Verification items for the finished model (mm, model axes). A direction names the side the tool comes from. Round coordinates to 2 decimals unless told otherwise and drop trailing zeros. Loops run counter-clockwise (first coordinate to the right, second up) from the corner with the lowest first, then second, coordinate; pieces in that order, holes last. Notation, with made-up numbers: M 43.25,57 L 99.25,57 A32 cw 99.25,89 Z; hole C -25.75,-23.75 d4. An arc over 180 degrees is marked long. One line per item, written item: value.
from build123d import *

# Parameters (mm, degrees)
F0_R     = 5
F0_R_2   = 2.5
F1_DEPTH = 13
F0_R_3   = 7.5
F2_DEPTH = 3
F4_DEPTH = 3
F3_R     = 7.5
F3_R_2   = 5
F3_R_3   = 0.5
F5_DEPTH = 3
F6_R     = 1.425
F7_DEPTH = 25


with BuildPart() as f1:
    # F0 (on Front) → F1 (new body)
    with BuildSketch(Plane.XZ):
        Circle(F0_R)
        Circle(F0_R_2, mode=Mode.SUBTRACT)
    extrude(amount=F1_DEPTH)

    # F0 (on Front) → F2 (join)
    with BuildSketch(Plane.XZ):
        Circle(F0_R_3)
        Circle(F0_R, mode=Mode.SUBTRACT)
    extrude(amount=-F2_DEPTH)

    # F4 (add): a face of the model
    f4_faces = [f1.faces().sort_by_distance(p)[0] for p in [
        (-4.8585786438, 0, 0),
    ]]
    extrude(f4_faces, amount=F4_DEPTH)

    # F3 (on face) → F5 (join)
    with BuildSketch(Plane.XZ.offset(13)):
        Circle(F3_R)
        Circle(F3_R_2, mode=Mode.SUBTRACT)
        with Locations((5.9560983991, 0.7244942103)):
            Circle(F3_R_3, mode=Mode.SUBTRACT)
        with Locations((4.9608234595, 3.3749415703)):
            Circle(F3_R_3, mode=Mode.SUBTRACT)
    extrude(amount=-F5_DEPTH)

    # F6 (on Right) → F7 (cut)
    with BuildSketch(Plane.YZ):
        with Locations((-5, 0)):
            Circle(F6_R)
    extrude(amount=-F7_DEPTH, mode=Mode.SUBTRACT)


solid = f1.part
(1) Thickness scan on L1, parallel to Y at x = -4, z = 5.5; L2, parallel to Z at x = 0, y = -9; L3, parallel to Y at x = -4.25, z = -0.5. Record the ranges inside material, lowest first. Write a range as from..to.
Completed:
L1: y = -13..-10, 0..3
L2: z = -5..-2.5, 2.5..5
L3: y = -13..-6.33, -3.67..3
(2) Depth check by flat-ended pin: pin 1 Ø1 at (y, z) = (-11, 1) entering from +X; pin 2 Ø4 at (x, y) = (-3, -9.5) entering from -Z; pin 3 Ø3.5 at (y, z) = (-5, 0) entering from -X. Enter the tip coordinate at first touch or a pass-through.
Completed:
pin 1: stops at x = 7.48
pin 2: stops at z = -7.42
pin 3: stops at x = -5
(3) Sectioned sample at D-D on y = 1.25. Enter the section's corners in (x, z).
Completed:
outline: C 0,0 d15; hole C 0,0 d5
(4) Sectioned sample at C-C on z = 0. Enter the section's corners in (x, y) (3 decimals), and give its area (3 significant figures).
Completed:
outline: M -7.5,-13 L -2.5,-13 L -2.5,-6.425 L -5,-6.425 L -5,-10 L -7.5,-10 Z; M -7.5,0 L -5,0 L -5,-3.575 L -2.5,-3.575 L -2.5,3 L -7.5,3 Z; M 2.5,-13 L 7.5,-13 L 7.5,-10 L 5,-10 L 5,0 L 7.5,0 L 7.5,3 L 2.5,3 Z
area: 103 mm^2
(5) Sectioned sample at B-B on z = -2.25. Enter the section's corners in (x, y), and give its area (3 significant figures).
Completed:
outline: M -7.15,-13 L -1.09,-13 L -1.09,3 L -7.15,3 L -7.15,0 L -4.47,0 L -4.47,-10 L -7.15,-10 Z; M 1.09,-13 L 7.15,-13 L 7.15,-10 L 4.47,-10 L 4.47,0 L 7.15,0 L 7.15,3 L 1.09,3 Z
area: 140 mm^2
(6) Tool access check on faces 5 (the face through (4.77, -4.93, 1.5)), 6 (the face through (-2, 3, 2)), 7 (the face through (-7.493, -11.521, 0.33)), 8 (the face through (6.433, -11.521, 0.875)), 9 (the face through (-3.506, -3.684, -0.546)). Record the directions out of +Z, -Z, +X, -X, +Y, -Y that give a thin tool (end or side, any length) a straight path to the whole face; none if there is none.
Completed:
face 5: none
face 6: +Z, -Z, +X, -X, +Y
face 7: +Y, -Y
face 8: -Y
face 9: -X
(7) Sectioned sample at A-A on x = 0. Enter the section's corners in (y, z).
Completed:
outline: M -13,-7.5 L -10,-7.5 L -10,-5 L 0,-5 L 0,-7.5 L 3,-7.5 L 3,-2.5 L -13,-2.5 Z; M -13,2.5 L 3,2.5 L 3,7.5 L 0,7.5 L 0,5 L -10,5 L -10,7.5 L -13,7.5 Z
(8) Mould release check, pull along X, two halves, no side actions. Record for faces 1 (the face through (5.42, -11.52, 3.18)), 2 (the face through (2, 0, -5)), 3 (the face through (2.385, -4.888, 0.751)), 4 (the face through (-7.493, 1.479, 0.33)): +X half, -X half, draft (parallel to the pull), parting line (faces both ways), or undercut.
Completed:
face 1: undercut
face 2: draft
face 3: undercut
face 4: parting line
